For this review, take the finished solid that the model builds, in its own axes (mm). A direction names the side the tool comes from. Coordinates: 2 decimals unless noted, no trailing zeros. Loops run counter-clockwise (first coordinate to the right, second up) from the corner with the lowest first, then second, coordinate; pieces in that order, holes last. Notation, with made-up numbers: (83.5, -1) - (116.5, -1) arc R26 cw to (116.5, 13) - close; hole circle Ø1 at (-35, -15). An arc over 180 degrees is marked (long way). One line per item, written item: value. Start each with the question number.
1. Insertion check: pin 1 (1.8 mm diameter, centred on x = -98.5, y = 2, fed in from -Z); pin 2 (3 mm diameter, centred on y = 2.5, z = 22.5, fed in from +X); pin 3 (1.8 mm diameter, centred on x = -143, y = 3.5, fed in from -Z). Each pin has a flat end and moves straight along its axis. Give the tip position at first contact, or say it passes through.
2. The part is to be moulded in two halves that separate along X. For faces 4 (the face through (-13.559, 3, 22)), 5 (the face through (100.3, 2.958, 27.867)), 6 (the face through (-143, 3, 19.02)), say which applies: released by +X, released by -X, zero draft, split by the parting line, or undercut.
3. Take a section at A-A, the plane z = -34. State the section outline as (x, y) points, and give its area (3 significant figures).
4. Take a section at B-B, the plane x = 1. State the section outline as (y, z) points.
5. For faces 1 (the face through (-123.009, 3, 15)), 2 (the face through (-100, 3, 4.97)), 3 (the face through (-84.559, 3, 22)), list the 3-axis set-ups (+Z, -Z, +X, -X, +Y, -Y) from which the entire face can be reached by the end or side of a thin tool; tool diameter is ignored.
6. Take a section at C-C, the plane y = 3.8. Count the separate pieces of the cut face and the enclosed holes in it, and give its area (3 significant figures).
7. To check wall thickness, follow line 1 (X direction, y = 2.85, z = 14); line 2 (X direction, y = 5.35, z = 9); line 3 (X direction, y = 0.3, z = -37). State the ranges of each line that lie inside material, in increasing order. Write a range as from..to.
```python
from build123d import *

# Parameters (mm, degrees)
SKETCH_1_R      = 1.55
SKETCH_1_W      = 10
SKETCH_1_H      = 6.1
EXTRUDE_1_DEPTH = 6


with BuildPart() as part:
    # Эскиз1 → Бобышка-Вытянуть1 (new body)
    with BuildSketch(Plane(origin=(0, 0, 0), x_dir=(1, 0, 0), z_dir=(0, 1, 0))):
        with BuildLine():
            Line((33.891038961, -17.86953047), (32.691038961, -17.86953047))
            Line((32.691038961, -17.86953047), (32.691038961, -20.06953047))
            Line((32.691038961, -20.06953047), (33.891038961, -20.06953047))
            Line((33.891038961, -20.06953047), (33.891038961, -21.56953047))
            Line((33.891038961, -21.56953047), (36.991038961, -21.56953047))
            Line((36.991038961, -21.56953047), (36.991038961, -20.06953047))
            Line((36.991038961, -20.06953047), (38.191038961, -20.06953047))
            Line((38.191038961, -20.06953047), (38.191038961, -17.86953047))
            Line((38.191038961, -17.86953047), (36.991038961, -17.86953047))
            Line((36.991038961, -17.86953047), (36.991038961, -11.06953047))
            Line((36.991038961, -11.06953047), (74.441038961, -11.06953047))
            ThreePointArc((74.441038961, -11.06953047), (87.168961022, -5.797452531), (92.441038961, 6.93046953))
            Line((92.441038961, 6.93046953), (92.441038961, 36.93046953))
            ThreePointArc((92.441038961, 36.93046953), (93.612611836, 39.758896655), (96.441038961, 40.93046953))
            Line((96.441038961, 40.93046953), (107.441038961, 40.93046953))
            Line((107.441038961, 40.93046953), (107.441038961, 14.48046953))
            Line((107.441038961, 14.48046953), (101.341038961, 14.48046953))
            Line((101.341038961, 14.48046953), (101.341038961, -0.61953047))
            Line((101.341038961, -0.61953047), (107.441038961, -0.61953047))
            Line((107.441038961, -0.61953047), (107.441038961, -19.06953047))
            Line((107.441038961, -19.06953047), (101.441038961, -19.06953047))
            Line((101.441038961, -19.06953047), (101.441038961, -25.06953047))
            ThreePointArc((101.441038961, -25.06953047), (100.269466086, -27.897957594), (97.441038961, -29.06953047))
            Line((97.441038961, -29.06953047), (-144.559273551, -29.06953047))
            ThreePointArc((-144.559273551, -29.06953047), (-147.369967416, -27.915580364), (-148.558961039, -25.11953047))
            Line((-148.558961039, -25.11953047), (-138.558961039, -25.11953047))
            Line((-138.558961039, -25.11953047), (-138.558961039, -19.01953047))
            Line((-138.558961039, -19.01953047), (-148.558961039, -19.01953047))
            Line((-148.558961039, -19.01953047), (-148.558961039, -15.06953047))
            ThreePointArc((-148.558961039, -15.06953047), (-147.387388164, -12.241103345), (-144.558961039, -11.06953047))
            Line((-144.558961039, -11.06953047), (-126.108961039, -11.06953047))
            Line((-126.108961039, -11.06953047), (-126.108961039, -17.86953047))
            Line((-126.108961039, -17.86953047), (-127.308961039, -17.86953047))
            Line((-127.308961039, -17.86953047), (-127.308961039, -20.06953047))
            Line((-127.308961039, -20.06953047), (-126.108961039, -20.06953047))
            Line((-126.108961039, -20.06953047), (-126.108961039, -21.56953047))
            Line((-126.108961039, -21.56953047), (-123.008961039, -21.56953047))
            Line((-123.008961039, -21.56953047), (-123.008961039, -20.06953047))
            Line((-123.008961039, -20.06953047), (-121.808961039, -20.06953047))
            Line((-121.808961039, -20.06953047), (-121.808961039, -17.86953047))
            Line((-121.808961039, -17.86953047), (-123.008961039, -17.86953047))
            Line((-123.008961039, -17.86953047), (-123.008961039, -11.06953047))
            Line((-123.008961039, -11.06953047), (-104.808961039, -11.06953047))
            Line((-104.808961039, -11.06953047), (-104.558961039, -4.96953047))
            Line((-104.558961039, -4.96953047), (-94.558961039, -4.96953047))
            Line((-94.558961039, -4.96953047), (-94.308961039, -11.06953047))
            Line((-94.308961039, -11.06953047), (5.191038961, -11.06953047))
            Line((5.191038961, -11.06953047), (5.441038961, -4.96953047))
            Line((5.441038961, -4.96953047), (15.441038961, -4.96953047))
            Line((15.441038961, -4.96953047), (15.691038961, -11.06953047))
            Line((15.691038961, -11.06953047), (33.891038961, -11.06953047))
            Line((33.891038961, -11.06953047), (33.891038961, -17.86953047))
        make_face()
        with Locations((104.441038961, 26.93046953)):
            Circle(SKETCH_1_R, mode=Mode.SUBTRACT)
        with Locations((104.441038961, -13.06953047)):
            Circle(SKETCH_1_R, mode=Mode.SUBTRACT)
        with Locations((-106.558961039, -22.06953047)):
            Circle(SKETCH_1_R, mode=Mode.SUBTRACT)
        with Locations((-38.558961039, -22.06953047)):
            Circle(SKETCH_1_R, mode=Mode.SUBTRACT)
        with Locations((21.441038961, -22.06953047)):
            Circle(SKETCH_1_R, mode=Mode.SUBTRACT)
        with Locations((89.441038961, -22.06953047)):
            Circle(SKETCH_1_R, mode=Mode.SUBTRACT)
        with Locations((-89.558961039, -22.06953047)):
            Rectangle(SKETCH_1_W, SKETCH_1_H, mode=Mode.SUBTRACT)
        with Locations((72.441038961, -22.06953047)):
            Rectangle(SKETCH_1_W, SKETCH_1_H, mode=Mode.SUBTRACT)
        with Locations((-8.558961039, -22.06953047)):
            Rectangle(SKETCH_1_W, SKETCH_1_H, mode=Mode.SUBTRACT)
    extrude(amount=EXTRUDE_1_DEPTH)


solid = part.part
```
Solutions:
1. pin 1: z = 4.97
1. pin 2: x = 101.44
1. pin 3: z = 11.07
2. face 4: undercut
2. face 5: released by +X
2. face 6: zero draft
3. outline: (92.44, 0) - (107.44, 0) - (107.44, 6) - (92.44, 6) - close
3. area: 90.0 mm2
4. outline: (0, 11.07) - (6, 11.07) - (6, 29.07) - (0, 29.07) - close
5. face 1: -Z, +Y, -Y
5. face 2: -Z, -X, +Y, -Y
5. face 3: +Y, -Y
6. separate pieces: 1
6. enclosed holes: 9
6. area: 5,050 mm2
7. line 1: -148.41..-126.11, -123.01..33.89, 36.99..103.2, 105.68..107.44
7. line 2: -104.72..-94.39, 5.28..15.61, 82.82..107.44
7. line 3: 92.44..107.44
